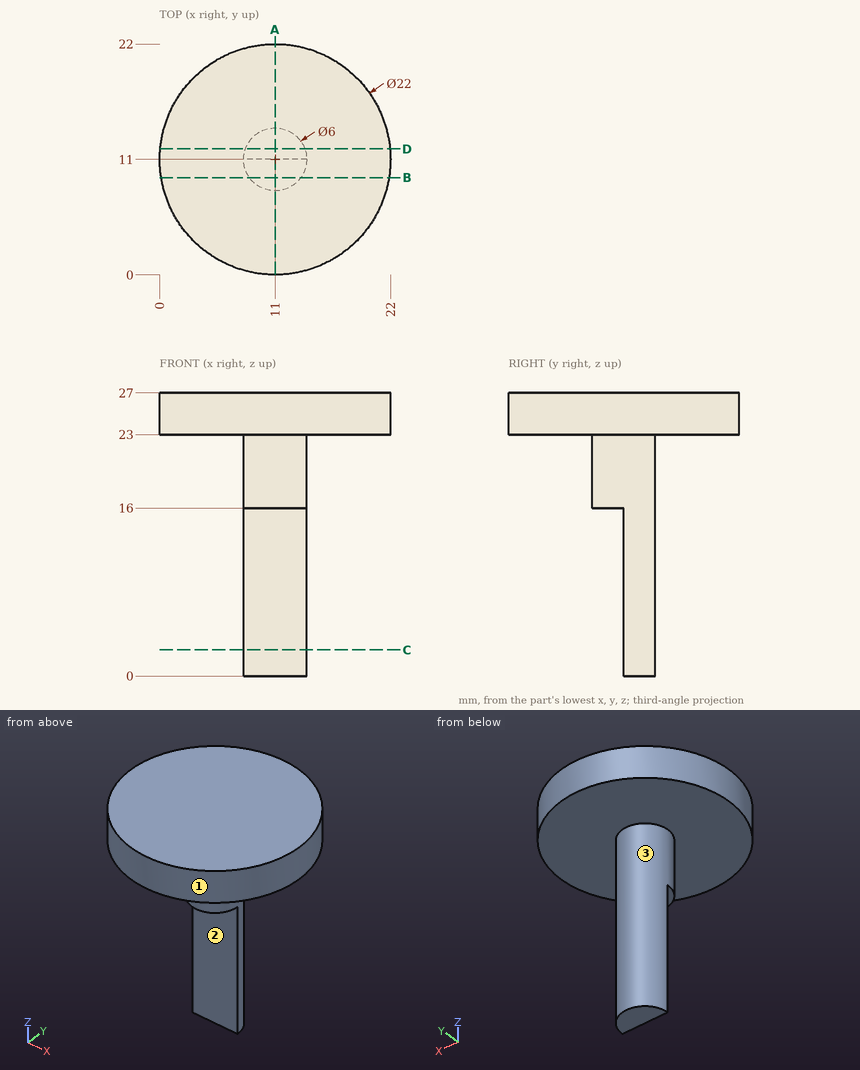
Input: dimensioned drawing with shaded views. Units: mm. Origin: part minimum x, y, z. A direction names the side the tool comes from. Round coordinates to 2 decimals unless told otherwise and drop trailing zeros. Loops run counter-clockwise (first coordinate to the right, second up) from the corner with the lowest first, then second, coordinate; pieces in that order, holes last. Notation, with made-up numbers: M 67.5,15.5 L 86.5,15.5 A24 ccw 86.5,38.5 Z; hole C -16,40.25 d10. An arc over 180 degrees is marked long. Answer in a Markdown table with one row per item. Add a question column.
1. Section C-C (z = 2.5). Output: boundary loops of the cut face in (x, y).
2. Section B-B (y = 9.25). Output: boundary loops of the cut face in (x, z), and give its area (3 significant figures).
3. Set-up query: the marked faces 1, 2 and 3. Return all of +Z, -Z, +X, -X, +Y, -Y with unobstructed straight access to the full face (end or side cutting, diameter ignored); none if empty.
4. Ray query, probe 1 along Z at (x, y) = (11.5, 16.25); probe 2 along Z at (x, y) = (12.5, 9); probe 3 along X at (y, z) = (12, 11.75). Return the intervals inside material, ascending.
5. Section D-D (y = 12). Output: boundary loops of the cut face in (x, z).
6. Section A-A (x = 11). Output: boundary loops of the cut face in (y, z), and give its area (3 significant figures).
7. Contact query for flat-ended pins moving along their axis: pin 1 (1.5 mm diameter, centred on x = 9.5, y = 9, fed in from -Z); pin 2 (4 mm diameter, centred on y = 14, z = 12, fed in from -X); pin 3 (3 mm diameter, centred on x = 11, z = 4, fed in from -Y). Output: stop coordinate, or through.
Values follow:
| question | item | result |
|---|---|---|
| 1 | outline | M 8,11 L 14,11 A3 ccw Z |
| 2 | outline | M 0.14,23 L 8.56,23 L 8.56,16 L 13.44,16 L 13.44,23 L 21.86,23 L 21.86,27 L 0.14,27 Z |
| 2 | area | 121 mm^2 |
| 3 | face 1 | +Z, -Z |
| 3 | face 2 | -Z, +X, -X, -Y |
| 3 | face 3 | -Z |
| 4 | probe 1 | 23 to 27 |
| 4 | probe 2 | 16 to 27 |
| 4 | probe 3 | 8.17 to 13.83 |
| 5 | outline | M 0.05,23 L 8.17,23 L 8.17,0 L 13.83,0 L 13.83,23 L 21.95,23 L 21.95,27 L 0.05,27 Z |
| 6 | outline | M 0,23 L 8,23 L 8,16 L 11,16 L 11,0 L 14,0 L 14,23 L 22,23 L 22,27 L 0,27 Z |
| 6 | area | 178 mm^2 |
| 7 | pin 1 | z = 16 |
| 7 | pin 2 | x = 8.17 |
| 7 | pin 3 | y = 11 |
